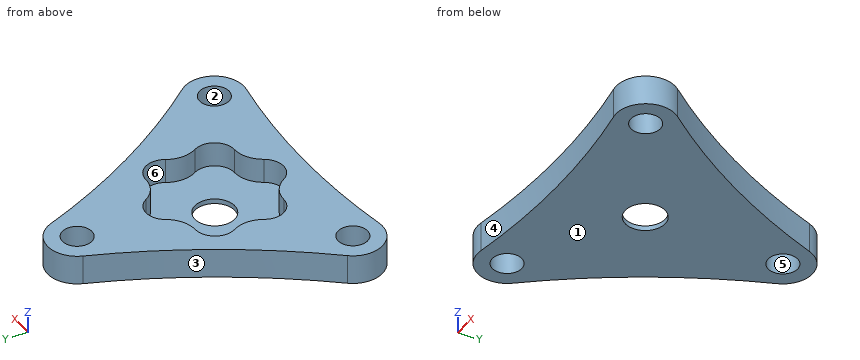
Autodesk Inventor part; units mm, degrees
ref_plane "YZ Plane" through (0, 0, 0) normal (1, 0, 0) x (0, 1, 0)
ref_plane "XZ Plane" through (0, 0, 0) normal (0, 1, 0) x (-1, 0, 0)
ref_plane "XY Plane" through (0, 0, 0) normal (0, 0, 1) x (1, 0, 0)
sketch "スケッチ1" plane through (0, 0, 0) normal (0, 0, 1) x (1, 0, 0)
  circle A0 centre (0, 0) radius 18.25
  circle A1 centre (0, 0) radius 17
  line L0 (0, 14) -> (12.1244, -7) construction
  line L1 (12.1244, -7) -> (-12.1244, -7) construction
  line L2 (-12.1244, -7) -> (0, 14) construction
  circle A2 centre (0, 14) radius 1.5
  circle A3 centre (-12.1244, -7) radius 1.5
  circle A4 centre (12.1244, -7) radius 1.5
  circle A5 centre (0, 14) radius 3
  circle A6 centre (-12.1244, -7) radius 3
  circle A7 centre (12.1244, -7) radius 3
  circle A8 centre (0, 0) radius 8 construction
  circle A9 centre (0, 0) radius 7 construction
  line L3 (0, 7) -> (6.0622, 3.5) construction
  line L4 (6.0622, 3.5) -> (6.0622, -3.5) construction
  line L5 (6.0622, -3.5) -> (0, -7) construction
  line L6 (0, -7) -> (-6.0622, -3.5) construction
  line L7 (-6.0622, -3.5) -> (-6.0622, 3.5) construction
  line L8 (-6.0622, 3.5) -> (0, 7) construction
  arc A10 (1.7321, 6) -> (-1.7321, 6) centre (0, 5) ccw
  arc A11 (-4.3301, 4.5) -> (-6.0622, 1.5) centre (-4.3301, 2.5) ccw
  arc A12 (-6.0622, -1.5) -> (-4.3301, -4.5) centre (-4.3301, -2.5) ccw
  arc A13 (-1.7321, -6) -> (1.7321, -6) centre (0, -5) ccw
  arc A14 (4.3301, -4.5) -> (6.0622, -1.5) centre (4.3301, -2.5) ccw
  arc A15 (6.0622, 1.5) -> (4.3301, 4.5) centre (4.3301, 2.5) ccw
  arc A16 (1.7321, 6) -> (4.3301, 4.5) centre (4.3301, 7.5) ccw
  arc A17 (-4.3301, 4.5) -> (-1.7321, 6) centre (-4.3301, 7.5) ccw
  arc A18 (-6.0622, -1.5) -> (-6.0622, 1.5) centre (-8.6603, 0) ccw
  arc A19 (-1.7321, -6) -> (-4.3301, -4.5) centre (-4.3301, -7.5) ccw
  arc A20 (4.3301, -4.5) -> (1.7321, -6) centre (4.3301, -7.5) ccw
  arc A21 (6.0622, 1.5) -> (6.0622, -1.5) centre (8.6603, 0) ccw
  circle A22 centre (0, 0) radius 5.6603 construction
  arc A23 (-14.4416, -5.0946) -> (-2.8087, 15.0541) centre (-69.282, 40) ccw
  arc A24 (11.6328, -9.9595) -> (-11.6328, -9.9595) centre (0, -80) ccw
  arc A25 (2.8087, 15.0541) -> (14.4416, -5.0946) centre (69.282, 40) ccw
  circle A26 centre (0, 0) radius 9 construction
  circle A27 centre (0, 0) radius 2.025
  point P0 (-15.3265, -15.7621)
  point P1 (-6.0622, -3.5)
  point P2 (0, -7)
  point P3 (6.0622, -3.5)
  point P4 (6.0622, 3.5)
  point P5 (-1.7321, -6)
  point P6 (-4.3301, -4.5)
  point P7 (-6.0622, -1.5)
  point P8 (-6.0622, 1.5)
  point P9 (-4.3301, 4.5)
  point P10 (6.0622, 1.5)
  point P11 (6.0622, -1.5)
  point P12 (4.3301, -4.5)
  point P13 (1.7321, -6)
  point P14 (-11.6328, -9.9595)
  point P15 (11.6328, -9.9595)
  point P16 (14.4416, -5.0946)
  point P17 (2.8087, 15.0541)
  dimension "d4" = 6
  dimension "d5" = 6
  dimension "d13" = 14
  dimension "d0" = 34
  dimension "d1" = 3
  dimension "d2" = 3
  dimension "d3" = 3
  dimension "d6" = 6
  dimension "d7" = 14
  dimension "d12" = 16
  dimension "d14" = 360
  dimension "d15" = 360
  dimension "d16" = 11.3205
  dimension "d17" = 3
  dimension "d18" = 2
  dimension "d21" = 360
  dimension "d23" = 18
  dimension "d28" = 4.05
extrude "押し出し1" add sketch "スケッチ1" along normal blind 3 contours A5 | A7 | A6 | A25 A7 A24 A6 A23 A5
extrude "押し出し2" add sketch "スケッチ1" along normal blind 0.5 contours A16 A15 A21 A14 A20 A13 A19 A12 A18 A11 A17 A10
properties part number "m0.5z80接続部品" material "アルミニウム 2014-T4"
Build history of the part. All positions in model axes, mm. Face numbers are marked on the shaded views. A direction names the side the tool comes from. Round coordinates to 2 decimals unless told otherwise and drop trailing zeros. Loops run counter-clockwise (first coordinate to the right, second up) from the corner with the lowest first, then second, coordinate; pieces in that order, holes last.
Item 1: Pin check, flat tips, straight feed: P1, Ø3.5, axis at x = 0, y = 0, coming from the -Z side; P2, Ø1.5, axis at y = 1, z = 1.5, coming from the -X side. Stop position of each tip, or through.
Item 2: Drill centre lines: line 1 along Y through (x, z) = (0, 0.45) (3 decimals); line 2 along X through (y, z) = (6.5, 1.5); line 3 along X through (y, z) = (1.5, 2.75). Where is each one in solid material? Low to high.
Item 3: Two-plate mould, pull along X, no slides. Class the marked faces 1, 2, 3 and 4: released by +X, released by -X, zero draft, split by the parting line, or undercut.
Item 4: Saw through at B-B (y = 14). List the corners of the cut face in (x, z).
Item 5: Saw through at A-A (x = 0). List the corners of the cut face in (y, z) (3 decimals), then the cut area to 3 significant figures.
Item 6: Saw through at C-C (z = 1). List the corners of the cut face in (x, y), then the cut area to 3 significant figures.
Item 7: Which spindle directions (+Z, -Z, +X, -X, +Y, -Y) get a long thin tool onto all of the face, cutting with end or side? Do the marked faces 5 and 6. Say none if no direction does.
Item 8: Saw through at D-D (x = -11). List the corners of the cut face in (y, z), then the cut area to 3 significant figures.
Worked answers:
1. P1: passes through
1. P2: stops at x = -10.45
2. line 1: y = -9 to -2.025, 2.025 to 12.5, 15.5 to 17
2. line 2: x = -6.68 to -1.32, 1.32 to 6.68
2. line 3: x = -9.63 to -6.06, 6.06 to 9.63
3. face 1: zero draft
3. face 2: undercut
3. face 3: released by -X
3. face 4: undercut
4. outline: (-3.21, 0) - (-1.5, 0) - (-1.5, 3) - (-3.21, 3) - close; (1.5, 0) - (3.21, 0) - (3.21, 3) - (1.5, 3) - close
5. outline: (-9, 0) - (-2.025, 0) - (-2.025, 0.5) - (-7, 0.5) - (-7, 3) - (-9, 3) - close; (2.025, 0) - (12.5, 0) - (12.5, 3) - (7, 3) - (7, 0.5) - (2.025, 0.5) - close; (15.5, 0) - (17, 0) - (17, 3) - (15.5, 3) - close
5. area: 32.0 mm2
6. outline: (-14.44, -5.09) arc R3 ccw to (-11.63, -9.96) arc R71 cw to (11.63, -9.96) arc R3 ccw to (14.44, -5.09) arc R71 cw to (2.81, 15.05) arc R3 ccw to (-2.81, 15.05) arc R71 cw to start; hole circle Ø3 at (-12.12, -7); hole (-6.06, -1.5) arc R2 ccw to (-4.33, -4.5) arc R3 cw to (-1.73, -6) arc R2 ccw to (1.73, -6) arc R3 cw to (4.33, -4.5) arc R2 ccw to (6.06, -1.5) arc R3 cw to (6.06, 1.5) arc R2 ccw to (4.33, 4.5) arc R3 cw to (1.73, 6) arc R2 ccw to (-1.73, 6) arc R3 cw to (-4.33, 4.5) arc R2 ccw to (-6.06, 1.5) arc R3 cw to start; hole circle Ø3 at (0, 14); hole circle Ø3 at (12.12, -7)
6. area: 306 mm2
7. face 5: +Z, -Z
7. face 6: +Z
8. outline: (-9.86, 0) - (-7.99, 0) - (-7.99, 3) - (-9.86, 3) - close; (-6.01, 0) - (-0.55, 0) - (-0.55, 3) - (-6.01, 3) - close
8. area: 22.0 mm2
